CAD build for the part. Positions are in the model's coordinates, mm. Face numbers are marked on the shaded views. A direction names the side the tool comes from. Coordinates: 2 decimals unless noted, no trailing zeros. Write each loop counter-clockwise with the first axis right and the second up, starting at its lowest first coordinate (ties: lowest second). Pieces come first, ordered by that corner, then holes. Notation, with made-up numbers: M 26.25,80 L 78.25,80 A21 cw 78.25,97 Z; hole C 23.5,45.25 d11. An arc over 180 degrees is marked long. Put each result on its own line as item: value. Start each with the question number.
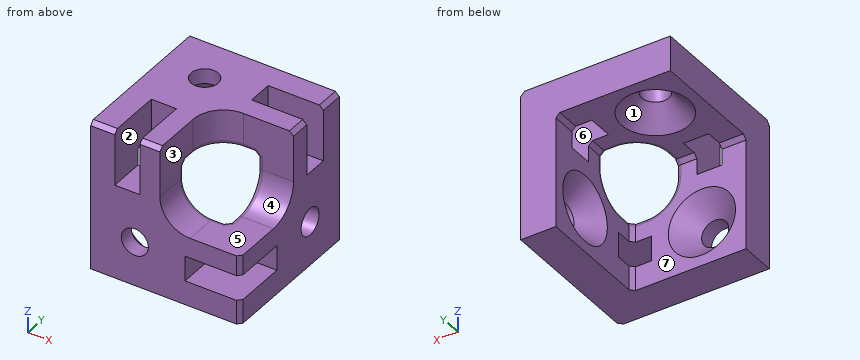
```python
from build123d import *

# Parameters (mm, degrees)
ESQUISSE1_W                                        = 16
ESQUISSE1_H                                        = 16
BOSS_EXTRU_1_DEPTH                                 = 16
COQUE2_T                                           = -3.5
ESQUISSE2_W                                        = 2.5
ESQUISSE2_H                                        = 5.5
ESQUISSE2_W_2                                      = 5.5
ESQUISSE2_H_2                                      = 2.5
ENL_V_MAT_EXTRU_1_DEPTH                            = 5.5
ESQUISSE3_W                                        = 5.5
ESQUISSE3_H                                        = 2.5
ENL_V_MAT_EXTRU_2_DEPTH                            = 5.5
ENL_V_MAT_EXTRU_3_DEPTH                            = 3.5
ENL_V_MAT_EXTRU_4_DEPTH                            = 3.5
ENL_V_MAT_EXTRU_5_DEPTH                            = 3.5
FRAISAGE_POUR_VIS_T_TE_FRAIS_E_M2_51_D             = 2.7
FRAISAGE_POUR_VIS_T_TE_FRAIS_E_M2_51_CSINK_D       = 6.7
FRAISAGE_POUR_VIS_T_TE_FRAIS_E_M2_51_CSINK_ANGLE   = 90
FRAISAGE_POUR_VIS_T_TE_FRAIS_E_M2_51_O_D           = 2.7
FRAISAGE_POUR_VIS_T_TE_FRAIS_E_M2_51_O_CSINK_D     = 6.7
FRAISAGE_POUR_VIS_T_TE_FRAIS_E_M2_51_O_CSINK_ANGLE = 90
FRAISAGE_POUR_VIS_T_TE_FRAIS_E_M2_2_D              = 2.7
FRAISAGE_POUR_VIS_T_TE_FRAIS_E_M2_2_CSINK_D        = 6.7
FRAISAGE_POUR_VIS_T_TE_FRAIS_E_M2_2_CSINK_ANGLE    = 90
ENL_V_MAT_EXTRU_6_DEPTH                            = 1.1
ENL_V_MAT_EXTRU_7_DEPTH                            = 1.1
ENL_V_MAT_EXTRU_8_DEPTH                            = 1.1
CHANFREIN1_SIZE                                    = 0.4
CONG_1_R                                           = 0.4


with BuildPart() as part:
    # Esquisse1 → Boss.-Extru.1 (new body)
    with BuildSketch(Plane(origin=(0, 0, 0), x_dir=(1, 0, 0), z_dir=(0, 1, 0))):
        Rectangle(ESQUISSE1_W, ESQUISSE1_H)
    extrude(amount=BOSS_EXTRU_1_DEPTH)

    # Coque2
    coque2_openings = [part.faces().sort_by_distance(p)[0] for p in [
        (0, 16, 0),
        (-8, 8, 0),
        (0, 8, -8),
    ]]
    offset(amount=COQUE2_T, openings=coque2_openings, kind=Kind.INTERSECTION)

    # Esquisse2 → Enlèv. mat.-Extru.1 (cut)
    with BuildSketch(Plane.XZ):
        with Locations((-3.25, 5.25)):
            Rectangle(ESQUISSE2_W, ESQUISSE2_H)
        with Locations((5.25, -3.25)):
            Rectangle(ESQUISSE2_W_2, ESQUISSE2_H_2)
    extrude(amount=-ENL_V_MAT_EXTRU_1_DEPTH, mode=Mode.SUBTRACT)

    # Esquisse3 → Enlèv. mat.-Extru.2 (cut)
    with BuildSketch(Plane.XY.offset(8)):
        with Locations((5.25, 11.25)):
            Rectangle(ESQUISSE3_W, ESQUISSE3_H)
    extrude(amount=-ENL_V_MAT_EXTRU_2_DEPTH, mode=Mode.SUBTRACT)

    # Esquisse7 → Enlèv. mat.-Extru.3 (cut)
    with BuildSketch(Plane.XZ):
        with BuildLine():
            Line((3, 0), (8, 0))
            Line((8, 0), (8, 8))
            Line((8, 8), (0, 8))
            Line((0, 8), (0, 3))
            ThreePointArc((0, 3), (0.878679656, 0.878679656), (3, 0))
        make_face()
    extrude(amount=-ENL_V_MAT_EXTRU_3_DEPTH, mode=Mode.SUBTRACT)

    # Esquisse8 → Enlèv. mat.-Extru.4 (cut)
    with BuildSketch(Plane.XY.offset(8)):
        with BuildLine():
            Line((3, 8), (8, 8))
            Line((8, 8), (8, 0))
            Line((8, 0), (0, 0))
            Line((0, 0), (0, 5))
            ThreePointArc((0, 5), (0.878679656, 7.121320344), (3, 8))
        make_face()
    extrude(amount=-ENL_V_MAT_EXTRU_4_DEPTH, mode=Mode.SUBTRACT)

    # Esquisse9 → Enlèv. mat.-Extru.5 (cut)
    with BuildSketch(Plane(origin=(8, 0, 0), x_dir=(0, 0, -1), z_dir=(1, 0, 0))):
        with BuildLine():
            Line((-3, 8), (-8, 8))
            Line((-8, 8), (-8, 0))
            Line((-8, 0), (0, 0))
            Line((0, 0), (0, 5))
            ThreePointArc((0, 5), (-0.878679656, 7.121320344), (-3, 8))
        make_face()
    extrude(amount=-ENL_V_MAT_EXTRU_5_DEPTH, mode=Mode.SUBTRACT)

    # Fraisage pour vis à tête fraisée M2.51 (through all)
    with Locations(Plane(origin=(4.5, 10.5, -2.5), x_dir=(0, 0, -1), z_dir=(-1, 0, 0))):
        with Locations((0, 0)):
            CounterSinkHole(FRAISAGE_POUR_VIS_T_TE_FRAIS_E_M2_51_D / 2, FRAISAGE_POUR_VIS_T_TE_FRAIS_E_M2_51_CSINK_D / 2, counter_sink_angle=FRAISAGE_POUR_VIS_T_TE_FRAIS_E_M2_51_CSINK_ANGLE)

    # Fraisage pour vis à tête fraisée M2.51 o (through all)
    with Locations(Plane(origin=(-2.5, 10.5, 4.5), x_dir=(-1, 0, 0), z_dir=(0, 0, -1))):
        with Locations((0, 0)):
            CounterSinkHole(FRAISAGE_POUR_VIS_T_TE_FRAIS_E_M2_51_O_D / 2, FRAISAGE_POUR_VIS_T_TE_FRAIS_E_M2_51_O_CSINK_D / 2, counter_sink_angle=FRAISAGE_POUR_VIS_T_TE_FRAIS_E_M2_51_O_CSINK_ANGLE)

    # Fraisage pour vis _ t_te frais_e M2. 2 (through all)
    with Locations(Plane(origin=(-2.5, 3.5, -2.5), x_dir=(0, 0, 1), z_dir=(0, 1, 0))):
        with Locations((0, 0)):
            CounterSinkHole(FRAISAGE_POUR_VIS_T_TE_FRAIS_E_M2_2_D / 2, FRAISAGE_POUR_VIS_T_TE_FRAIS_E_M2_2_CSINK_D / 2, counter_sink_angle=FRAISAGE_POUR_VIS_T_TE_FRAIS_E_M2_2_CSINK_ANGLE)

    # Esquisse10 → Enlèv. mat.-Extru.6 (cut)
    with BuildSketch(Plane(origin=(0, 16, 0), x_dir=(1, 0, 0), z_dir=(0, 1, 0))):
        Polygon((4.5, 8), (4.5, -4.5), (-8, -4.5), (-8, -8), (8, -8), (8, 8), align=None)
    extrude(amount=-ENL_V_MAT_EXTRU_6_DEPTH, mode=Mode.SUBTRACT)

    # Esquisse11 → Enlèv. mat.-Extru.7 (cut)
    with BuildSketch(Plane(origin=(0, 0, -8), x_dir=(-1, 0, 0), z_dir=(0, 0, -1))):
        Polygon((-4.5, 14.9), (-8, 14.9), (-8, 0), (8, 0), (8, 3.5), (-4.5, 3.5), align=None)
    extrude(amount=-ENL_V_MAT_EXTRU_7_DEPTH, mode=Mode.SUBTRACT)

    # Esquisse13 → Enlèv. mat.-Extru.8 (cut)
    with BuildSketch(Plane.ZY.offset(8)):
        Polygon((-6.9, 3.5), (-6.9, 0), (8, 0), (8, 14.9), (4.5, 14.9), (4.5, 3.5), align=None)
    extrude(amount=-ENL_V_MAT_EXTRU_8_DEPTH, mode=Mode.SUBTRACT)

    # Chanfrein1
    chanfrein1_edges = [part.edges().sort_by_distance(p)[0] for p in [
        (4.5, 13.7, 4.5),
        (8, 13.7, 8),
        (-5.7, 3.5, 4.5),
        (-5.7, 0, 8),
        (4.5, 3.5, -5.7),
        (-1, 3.5, 4.5),
        (8, 0, -5.7),
        (-1, 0, 8),
        (4.5, 9, 4.5),
        (8, 9, 8),
        (4.5, 3.5, -1),
        (8, 0, -1),
    ]]
    chamfer(chanfrein1_edges, length=CHANFREIN1_SIZE)

    # Congé1
    cong_1_edges = [part.edges().sort_by_distance(p)[0] for p in [
        (0.878679656, 3.5, 0.878679656),
        (0, 4.45, 4.5),
        (0.878679656, 7.121320344, 4.5),
        (4.5, 8, 3.55),
        (4.5, 7.121320344, 0.878679656),
        (3.55, 8, 4.5),
        (4.5, 4.45, 0),
        (4.3, 8, 4.3),
        (0, 3.7, 4.3),
        (4.3, 3.7, 0),
        (0, 3.5, 3.55),
        (3.55, 3.5, 0),
    ]]
    fillet(cong_1_edges, radius=CONG_1_R)


solid = part.part
```
(1) Two-plate mould, pull along X, no slides. Class the marked faces 1, 2, 3 and 4: +X half, -X half, draft (parallel to the pull), parting line (faces both ways), or undercut.
(2) Slice it at C-C, the plane x = 3.5. Write the cut outline in (y, z), then the cut area to 3 significant figures.
(3) Slice it at A-A, the plane y = 1. Write the cut outline in (x, z).
(4) Which spindle directions (+Z, -Z, +X, -X, +Y, -Y) get a long thin tool onto all of the face, cutting with end or side? Do the marked faces 5, 6 and 7. Say none if no direction does.
(5) Slice it at B-B, the plane z = -2.5. Write the cut outline in (x, y).
(6) Drill centre lines: line 1 (X direction, y = 0.95, z = -2.5); line 2 (Z direction, x = 7, y = 3.25); line 3 (Y direction, x = -2.5, z = 7.05). Where is each one in solid material? Low to high. Write a range as [from, to].
(7) Drop flat-ended pins along their axis: pin 1 (3 mm diameter, centred on x = 4, z = 4.5, fed in from -Y); pin 2 (1.2 mm diameter, centred on y = 2.5, z = -3, fed in from +X); pin 3 (1.5 mm diameter, centred on x = 6.5, y = 1.5, fed in from +Z). Give the stop position or say it passes through.
(8) Slice it at D-D, the plane y = 4.75. Write the cut outline in (x, z), then the cut area to 3 significant figures.
Result set:
1. face 1: undercut
1. face 2: undercut
1. face 3: +X half
1. face 4: draft
2. outline: M 0,-6.9 L 3.5,-6.9 L 3.5,-4.5 L 0,-4.5 Z; M 0,-2 L 3.5,-2 L 3.5,-0.4 A0.4 ccw 3.1,0 L 0,0 Z; M 8,4.9 A0.4 ccw 8.4,4.5 L 10,4.5 L 10,8 L 8,8 Z; M 12.5,4.5 L 14.9,4.5 L 14.9,8 L 12.5,8 Z
2. area: 30.7 mm^2
3. outline: M -6.9,-6.9 L 8,-6.9 L 8,-4.5 L 2.5,-4.5 L 2.5,-2 L 8,-2 L 8,0 L 3,0 A3 cw 0,3 L 0,8 L -2,8 L -2,2.5 L -4.5,2.5 L -4.5,8 L -6.9,8 Z; hole C -2.5,-2.5 d2.7
4. face 5: +Z, +X, -Y
4. face 6: +Z, +X
4. face 7: -Z, -X, +Y
5. outline: M -6.9,0 L -3.85,0 L -3.85,1.5 L -5.85,3.5 L -6.9,3.5 Z; M -1.15,0 L 2.5,0 L 2.5,3.5 L 0.85,3.5 L -1.15,1.5 Z; M 4.5,5.5 L 8,5.5 L 8,9.15 L 6.5,9.15 L 4.5,7.15 Z; M 4.5,13.85 L 6.5,11.85 L 8,11.85 L 8,14.9 L 4.5,14.9 Z
6. line 1: x = [-6.9, -3.85], [-1.15, 2.5]
6. line 2: z = [-6.9, -4.5], [-2, 0]
6. line 3: y = [5.5, 9.15], [11.85, 14.9]
7. pin 1: stops at y = 7.97
7. pin 2: stops at x = 2.5
7. pin 3: stops at z = 0
8. outline: M -6.9,4.5 L -4.5,4.5 L -4.5,8 L -6.9,8 Z; M -2,4.5 L -0.4,4.5 A0.4 ccw 0,4.9 L 0,8 L -2,8 Z; M 4.5,-6.9 L 8,-6.9 L 8,-4.5 L 4.5,-4.5 Z; M 4.5,-2 L 8,-2 L 8,0 L 4.9,0 A0.4 ccw 4.5,-0.4 Z
8. area: 30.7 mm^2
